```python
from build123d import *

# Parameters (mm, degrees)
BOSS_EXTRUDE1_DEPTH   = 2.7686
BOSS_EXTRUDE2_START   = -2.7686
BOSS_EXTRUDE2_DEPTH   = 25.4
BOSS_EXTRUDE2_2_DEPTH = 25.4
SKETCH4_W             = 2.7686
SKETCH4_H             = 25.4
BOSS_EXTRUDE3_DEPTH   = 25.4
CUT_EXTRUDE1_DEPTH    = 2.7686
BOSS_EXTRUDE6_DEPTH   = 44.45
BOSS_EXTRUDE7_DEPTH   = 2.7686


with BuildPart() as part:
    # Sketch1 → Boss-Extrude1 (new body)
    with BuildSketch(Plane(origin=(0, 0, 0), x_dir=(1, 0, 0), z_dir=(0, 1, 0))):
        Polygon((0, 0), (44.45, 0), (123.825, -79.375), (-79.375, -79.375), align=None)
    extrude(amount=BOSS_EXTRUDE1_DEPTH)



with BuildPart() as body_2:
    # Sketch2 → Boss-Extrude2 (new body)
    with BuildSketch(Plane(origin=(0, 2.7686, 0), x_dir=(1, 0, 0), z_dir=(0, 1, 0)).offset(BOSS_EXTRUDE2_START)):
        Polygon((0, 0), (-79.375, -79.375), (-82.1436, -79.375), (-2.7686, 0), align=None)
    extrude(amount=BOSS_EXTRUDE2_DEPTH)


with BuildPart() as body_3:
    # Sketch2 → Boss-Extrude2 2 (new body)
    with BuildSketch(Plane(origin=(0, 2.7686, 0), x_dir=(1, 0, 0), z_dir=(0, 1, 0)).offset(BOSS_EXTRUDE2_START)):
        Polygon((44.45, 0), (47.2186, 0), (126.5936, -79.375), (123.825, -79.375), align=None)
    extrude(amount=BOSS_EXTRUDE2_2_DEPTH)


with BuildPart() as part_1:
    add(part.part)

    add(body_3.part)  # Boss-Extrude3 merges body 3
    # Sketch4 → Boss-Extrude3 (add)
    with BuildSketch(Plane(origin=(0, 0, 0), x_dir=(-1, 0, 0), z_dir=(0, 0, -1))):
        with Locations((-45.8343, 12.7)):
            Rectangle(SKETCH4_W, SKETCH4_H)
    extrude(amount=BOSS_EXTRUDE3_DEPTH)

    # Sketch5 → Cut-Extrude1 (cut)
    with BuildSketch(Plane(origin=(47.2186, 0, 0), x_dir=(0, 0, -1), z_dir=(1, 0, 0))):
        Polygon((17.186035514, 6.697089394), (0, 0), (25.4, 0), (25.4, 14.244871038), (25.4, 25.4), (0, 25.4), align=None)
    extrude(amount=-CUT_EXTRUDE1_DEPTH, mode=Mode.SUBTRACT)


    add(body_2.part)  # Boss-Extrude6 merges body 2
    # Sketch10 → Boss-Extrude6 (add)
    with BuildSketch(Plane.ZY.offset(-44.45)):
        with BuildLine():
            Line((-17.186035514, 6.697089394), (-15.298135688, 8.75161917))
            ThreePointArc((-15.298135688, 8.75161917), (-8.213243481, 4.317554379), (0, 2.7686))
            Line((0, 2.7686), (0, 0))
            Line((0, 0), (-17.186035514, 6.697089394))
        make_face()
    extrude(amount=BOSS_EXTRUDE6_DEPTH)

    # Sketch11 → Boss-Extrude7 (add)
    with BuildSketch(Plane.ZY):
        Polygon((0, 0), (0, 25.4), (-17.186035514, 6.697089394), align=None)
    extrude(amount=BOSS_EXTRUDE7_DEPTH)


solid = part_1.part
```
Verification items for the finished model (mm, model axes). A direction names the side the tool comes from. Coordinates: 2 decimals unless noted, no trailing zeros. Write each loop counter-clockwise with the first axis right and the second up, starting at its lowest first coordinate (ties: lowest second). Pieces come first, ordered by that corner, then holes. Notation, with made-up numbers: (-14, -36.5) - (35, -36.5) arc R28 cw to (35, 1.5) - close; hole circle Ø7 at (-28.5, 31.5). An arc over 180 degrees is marked (long way). One line per question, with ' | ' between items. Start each with the question number.
1. Material ranges on line 1 along X through (y, z) = (19, 0); line 2 along Y through (x, z) = (-22, 61); line 3 along X through (y, z) = (11.25, 37), recorded low to high.
2. Gauge pin test, flat ends, axial feed: P1, Ø5, axis at x = -27, y = 18, coming from the +Z side; P2, Ø12, axis at y = 13, z = -9, coming from the -X side; P3, Ø2, axis at x = 34.5, z = 65, coming from the +Y side. Record the tip position at first contact, or that the pin passes through.
3. Section check A-A (y = 20.5). Enter the section's corners in (x, z) (3 decimals).
4. Section check C-C (x = 36). Enter the section's corners in (y, z) (3 decimals).
5. Access from +Z, -Z, +X, -X, +Y, -Y to the whole of each face (thin tool, end or side, straight path). Record for faces 1 (the flat face through (24, 2.769, 48)), 2 (the flat face through (-2.769, 10, -5)), 3 (the flat face through (47.219, 10, -7)).
6. Draft check along X on faces 4 (the flat face through (-43.01, 12.52, 40.24)), 5 (the flat face through (-41, 25.4, 40)), 6 (the flat face through (44.45, 11, -6)). Enter one of: released by +X, released by -X, zero draft, split by the parting line, or undercut.
7. Section check B-B (z = 40). Enter the section's corners in (x, y).
8. Section check D-D (y = 11.5). Enter the section's corners in (x, z) (3 decimals), plus the area to 3 significant figures.
Computed values:
1) line 1: -2.77 to 0, 44.45 to 47.22 | line 2: 0 to 2.77 | line 3: -39.77 to -37, 81.45 to 84.22
2) P1: z = 29.5 | P2: x = -2.77 | P3: y = 2.77
3) outline: (-82.144, 79.375) - (-2.769, 0) - (-2.769, -4.503) - (0, -4.503) - (0, 0) - (-79.375, 79.375) - close; (44.45, -4.503) - (47.219, -4.503) - (47.219, 0) - (126.594, 79.375) - (123.825, 79.375) - (44.45, 0) - close
4) outline: (0, 0) - (6.697, -17.186) - (8.752, -15.298) arc R22.55 cw to (2.769, 0) - (2.769, 79.375) - (0, 79.375) - close
5) face 1: +Z, +Y | face 2: -Z, -X, +Y, -Y | face 3: -Z, +X, +Y, -Y
6) face 4: released by -X | face 5: zero draft | face 6: undercut
7) outline: (-42.77, 0) - (87.22, 0) - (87.22, 25.4) - (84.45, 25.4) - (84.45, 2.77) - (-40, 2.77) - (-40, 25.4) - (-42.77, 25.4) - close
8) outline: (-82.144, 79.375) - (-2.769, 0) - (-2.769, -12.773) - (0, -12.773) - (0, 0) - (-79.375, 79.375) - close; (44.45, -12.773) - (47.219, -12.773) - (47.219, 0) - (126.594, 79.375) - (123.825, 79.375) - (44.45, 0) - close | area: 510 mm²
